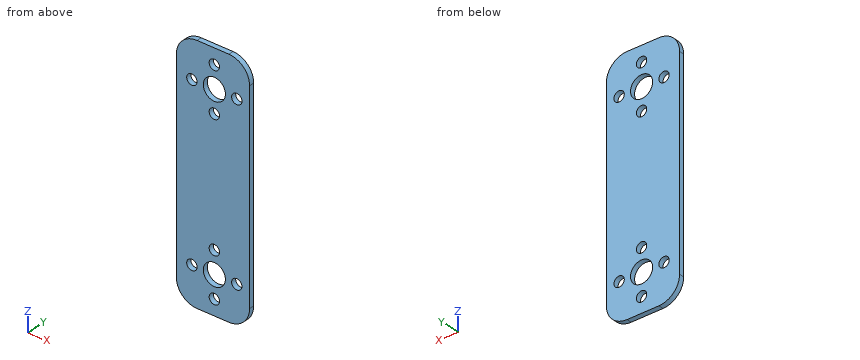
```python
from build123d import *

# Parameters (mm, degrees)
F0_R     = 1.905
F0_R_2   = 4.064
F1_DEPTH = 1.8542


with BuildPart() as f1:
    # F0 (on Front) → F1 (new body)
    with BuildSketch(Plane.XZ):
        with BuildLine():
            ThreePointArc((0, 33.470551), (-2.231846, 38.858705), (-7.62, 41.090551))
            Line((-7.62, 41.090551), (-19.304, 41.090551))
            ThreePointArc((-19.304, 41.090551), (-24.692154, 38.858705), (-26.924, 33.470551))
            Line((-26.924, 33.470551), (-26.924, -41.713449))
            ThreePointArc((-26.924, -41.713449), (-24.692154, -47.101602), (-19.304, -49.333449))
            Line((-19.304, -49.333449), (-7.62, -49.333449))
            ThreePointArc((-7.62, -49.333449), (-2.231846, -47.101602), (0, -41.713449))
            Line((0, -41.713449), (0, 33.470551))
        make_face()
        with Locations((-21.209, -35.363449)):
            Circle(F0_R, mode=Mode.SUBTRACT)
        with Locations((-12.954, -43.618449)):
            Circle(F0_R, mode=Mode.SUBTRACT)
        with Locations((-12.954, -35.363449)):
            Circle(F0_R_2, mode=Mode.SUBTRACT)
        with Locations((-12.954, -27.108449)):
            Circle(F0_R, mode=Mode.SUBTRACT)
        with Locations((-4.699, -35.363449)):
            Circle(F0_R, mode=Mode.SUBTRACT)
        with Locations((-21.209, 27.120551)):
            Circle(F0_R, mode=Mode.SUBTRACT)
        with Locations((-12.954, 18.865551)):
            Circle(F0_R, mode=Mode.SUBTRACT)
        with Locations((-12.954, 27.120551)):
            Circle(F0_R_2, mode=Mode.SUBTRACT)
        with Locations((-12.954, 35.375551)):
            Circle(F0_R, mode=Mode.SUBTRACT)
        with Locations((-4.699, 27.120551)):
            Circle(F0_R, mode=Mode.SUBTRACT)
    extrude(amount=F1_DEPTH)


solid = f1.part
```
CAD build for the part. Positions are in the model's coordinates, mm. Round coordinates to 2 decimals unless told otherwise and drop trailing zeros. Loops run counter-clockwise (first coordinate to the right, second up) from the corner with the lowest first, then second, coordinate; pieces in that order, holes last. Notation, with made-up numbers: M 69,-20.75 L 82,-20.75 A19 cw 82,10.25 Z; hole C 77.25,-20.5 d9. An arc over 180 degrees is marked long. Use a Markdown table: item, result. Add a question column.
(1) Drill centre lines: line 1 (Z direction, x = -10, y = -1.05); line 2 (Z direction, x = -15, y = -0.45); line 3 (X direction, y = -1.2, z = -36). Where is each one in solid material? Low to high.
(2) Cut at A-A (x = -5.25). Give the cut face in (y, z), and give its area (3 significant figures).
(3) Cut at C-C (x = -12.75). Give the cut face in (y, z).
(4) Cut at B-B (y = -1.3). State how many separate pieces and enclosed holes the cut face has, and give its area (3 significant figures).
(5) Cut at D-D (x = -16.25). Give the cut face in (y, z), and give its area (3 significant figures).
Geometry says:
| question | item | result |
|---|---|---|
| 1 | line 1 | z = -49.33 to -38.15, -32.57 to 24.33, 29.91 to 41.09 |
| 1 | line 2 | z = -49.33 to -38.87, -31.85 to 23.61, 30.63 to 41.09 |
| 1 | line 3 | x = -26.92 to -23, -19.41 to -16.97, -8.94 to -6.49, -2.9 to 0 |
| 2 | outline | M -1.85,-48.96 L 0,-48.96 L 0,-37.19 L -1.85,-37.19 Z; M -1.85,-33.54 L 0,-33.54 L 0,25.3 L -1.85,25.3 Z; M -1.85,28.94 L 0,28.94 L 0,40.71 L -1.85,40.71 Z |
| 2 | area | 153 mm² |
| 3 | outline | M -1.85,-49.33 L 0,-49.33 L 0,-45.51 L -1.85,-45.51 Z; M -1.85,-41.72 L 0,-41.72 L 0,-39.42 L -1.85,-39.42 Z; M -1.85,-31.3 L 0,-31.3 L 0,-29 L -1.85,-29 Z; M -1.85,-25.21 L 0,-25.21 L 0,16.97 L -1.85,16.97 Z; M -1.85,20.76 L 0,20.76 L 0,23.06 L -1.85,23.06 Z; M -1.85,31.18 L 0,31.18 L 0,33.48 L -1.85,33.48 Z; M -1.85,37.27 L 0,37.27 L 0,41.09 L -1.85,41.09 Z |
| 4 | separate pieces | 1 |
| 4 | enclosed holes | 10 |
| 4 | area | 2,190 mm² |
| 5 | outline | M -1.85,-49.33 L 0,-49.33 L 0,-37.74 L -1.85,-37.74 Z; M -1.85,-32.99 L 0,-32.99 L 0,24.74 L -1.85,24.74 Z; M -1.85,29.5 L 0,29.5 L 0,41.09 L -1.85,41.09 Z |
| 5 | area | 150 mm² |
